Verification items for the finished model (mm, model axes). Coordinates: 2 decimals unless noted, no trailing zeros. Write each loop counter-clockwise with the first axis right and the second up, starting at its lowest first coordinate (ties: lowest second). Pieces come first, ordered by that corner, then holes. Notation, with made-up numbers: (-12.5, 10.25) - (20.5, 10.25) arc R25 cw to (20.5, 25.25) - close; hole circle Ø10 at (41.5, -12). An arc over 180 degrees is marked (long way). Answer as CSV lines item,"result". Start each with the question number.
```python
from build123d import *

# Parameters (mm, degrees)
CROQUIS1_W              = 62.206373562
CROQUIS1_H              = 40
SALIENTE_EXTRUIR1_DEPTH = 5
CROQUIS9_R              = 3
CORTAR_EXTRUIR2_DEPTH   = 10


with BuildPart() as part:
    # Croquis1 → Saliente-Extruir1 (new body)
    with BuildSketch(Plane.XY):
        with Locations((69.078310012, 39.240002825)):
            Rectangle(CROQUIS1_W, CROQUIS1_H)
    extrude(amount=SALIENTE_EXTRUIR1_DEPTH)

    # Croquis9 → Cortar-Extruir2 (cut)
    with BuildSketch(Plane(origin=(0, 0, 0), x_dir=(-1, 0, 0), z_dir=(0, 0, -1))):
        with Locations((-94.181496793, 27.39443436)):
            Circle(CROQUIS9_R)
        with Locations((-94.181496793, 39.39443436)):
            Circle(CROQUIS9_R)
        with Locations((-94.181496793, 51.39443436)):
            Circle(CROQUIS9_R)
        with Locations((-43.975123231, 27.39443436)):
            Circle(CROQUIS9_R)
        with Locations((-43.975123231, 39.39443436)):
            Circle(CROQUIS9_R)
        with Locations((-43.975123231, 51.39443436)):
            Circle(CROQUIS9_R)
    extrude(amount=-CORTAR_EXTRUIR2_DEPTH, mode=Mode.SUBTRACT)


solid = part.part
```
1. Cross-section at C-C (y = 26). Record the cut outline in (x, z).
2. Draft check along X on faces 1 (the face through (46.972, 51.526, 2.465)), 2 (the face through (37.975, 39, 2)), 3 (the face through (100.181, 39, 2)), 4 (the face through (69, 40, 5)). Enter one of: pulls with the +X half, pulls with the -X half, needs draft (parallel to the pull), parting line crosses it, or undercut.
3. Scan lines: line 1 along X through (y, z) = (27.5, 2.6); line 2 along Y through (x, z) = (44.5, 3.75); line 3 along Y through (x, z) = (43.5, 0.6). Record each from-to range of solid material in increasing order. Write a range as from..to.
4. Depth check by flat-ended pin: P1, Ø8, axis at x = 43.98, y = 39.39, coming from the +Z side. Enter the tip coordinate at first touch or a pass-through.
5. Cross-section at B-B (z = 4.1). Record the cut outline in (x, y), and give its area (3 significant figures).
6. Cross-section at A-A (y = 37). Record the cut outline in (x, z).
Completed:
1,outline,"(37.98, 0) - (41.32, 0) - (41.32, 5) - (37.98, 5) - close; (46.63, 0) - (91.53, 0) - (91.53, 5) - (46.63, 5) - close; (96.84, 0) - (100.18, 0) - (100.18, 5) - (96.84, 5) - close"
2,face 1,"undercut"
2,face 2,"pulls with the -X half"
2,face 3,"pulls with the +X half"
2,face 4,"needs draft"
3,line 1,"x = 37.98..40.98, 46.97..91.18, 97.18..100.18"
3,line 2,"y = 19.24..24.44, 30.35..36.44, 42.35..48.44, 54.35..59.24"
3,line 3,"y = 19.24..24.43, 30.36..36.43, 42.36..48.43, 54.36..59.24"
4,P1,"stops at z = 5"
5,outline,"(37.98, 19.24) - (100.18, 19.24) - (100.18, 59.24) - (37.98, 59.24) - close; hole circle Ø6 at (43.98, 27.39); hole circle Ø6 at (43.98, 39.39); hole circle Ø6 at (43.98, 51.39); hole circle Ø6 at (94.18, 27.39); hole circle Ø6 at (94.18, 39.39); hole circle Ø6 at (94.18, 51.39)"
5,area,"2,320 mm2"
6,outline,"(37.98, 0) - (42.17, 0) - (42.17, 5) - (37.98, 5) - close; (45.78, 0) - (92.37, 0) - (92.37, 5) - (45.78, 5) - close; (95.99, 0) - (100.18, 0) - (100.18, 5) - (95.99, 5) - close"
